```python
from build123d import *

# Parameters (mm, degrees)
SKETCH2_R               = 20
SKETCH2_R_2             = 4
BOSS_EXTRUDE1_DEPTH     = 21
CUT_EXTRUDE2_REACH      = 79.672
SKETCH3_R               = 2.5
CUT_EXTRUDE3_REACH      = 79.672
CUT_EXTRUDE3_END_RADIUS = 20
SKETCH4_R               = 2


with BuildPart() as part:
    # Sketch1 → Revolve1 (revolve)
    with BuildSketch(Plane(origin=(0, 0, 0), x_dir=(0, 0, -1), z_dir=(1, 0, 0))):
        Polygon((0, 0), (0, 52), (4, 52), (4, 20), (25, 20), (25, 0), align=None)
    revolve(axis=Axis((0, 0, -25), (0, 0, 1)))

    # Sketch2 → Boss-Extrude1 (add)
    with BuildSketch(Plane.XY):
        with Locations(Location((0, 0, 0), (0, 0, 90))):
            Circle(SKETCH2_R)
        with Locations(Location((0, 0, 0), (0, 0, 180))):
            Circle(SKETCH2_R_2, mode=Mode.SUBTRACT)
    extrude(amount=BOSS_EXTRUDE1_DEPTH)

    # Sketch3 → Cut-Extrude2 (cut, up to next)
    with BuildSketch(Plane(origin=(0, 0, -4), x_dir=(-1, 0, 0), z_dir=(0, 0, -1)), mode=Mode.PRIVATE) as cut_extrude2_sk1:
        with Locations(Location((0, 40, 0), (0, 0, 90))):
            Circle(SKETCH3_R)
    cut_extrude2_tool1 = extrude(cut_extrude2_sk1.sketch, amount=-CUT_EXTRUDE2_REACH, mode=Mode.PRIVATE) & part.part
    # Sketch3 → Cut-Extrude2 (cut, up to next)
    with BuildSketch(Plane(origin=(0, 0, -4), x_dir=(-1, 0, 0), z_dir=(0, 0, -1)), mode=Mode.PRIVATE) as cut_extrude2_sk2:
        with Locations(Location((34.641016151, 20, 0), (0, 0, 90))):
            Circle(SKETCH3_R)
    cut_extrude2_tool2 = extrude(cut_extrude2_sk2.sketch, amount=-CUT_EXTRUDE2_REACH, mode=Mode.PRIVATE) & part.part
    # Sketch3 → Cut-Extrude2 (cut, up to next)
    with BuildSketch(Plane(origin=(0, 0, -4), x_dir=(-1, 0, 0), z_dir=(0, 0, -1)), mode=Mode.PRIVATE) as cut_extrude2_sk3:
        with Locations(Location((34.641016151, -20, 0), (0, 0, 90))):
            Circle(SKETCH3_R)
    cut_extrude2_tool3 = extrude(cut_extrude2_sk3.sketch, amount=-CUT_EXTRUDE2_REACH, mode=Mode.PRIVATE) & part.part
    # Sketch3 → Cut-Extrude2 (cut, up to next)
    with BuildSketch(Plane(origin=(0, 0, -4), x_dir=(-1, 0, 0), z_dir=(0, 0, -1)), mode=Mode.PRIVATE) as cut_extrude2_sk4:
        with Locations(Location((0, -40, 0), (0, 0, 90))):
            Circle(SKETCH3_R)
    cut_extrude2_tool4 = extrude(cut_extrude2_sk4.sketch, amount=-CUT_EXTRUDE2_REACH, mode=Mode.PRIVATE) & part.part
    # Sketch3 → Cut-Extrude2 (cut, up to next)
    with BuildSketch(Plane(origin=(0, 0, -4), x_dir=(-1, 0, 0), z_dir=(0, 0, -1)), mode=Mode.PRIVATE) as cut_extrude2_sk5:
        with Locations(Location((-34.641016151, -20, 0), (0, 0, 90))):
            Circle(SKETCH3_R)
    cut_extrude2_tool5 = extrude(cut_extrude2_sk5.sketch, amount=-CUT_EXTRUDE2_REACH, mode=Mode.PRIVATE) & part.part
    # Sketch3 → Cut-Extrude2 (cut, up to next)
    with BuildSketch(Plane(origin=(0, 0, -4), x_dir=(-1, 0, 0), z_dir=(0, 0, -1)), mode=Mode.PRIVATE) as cut_extrude2_sk6:
        with Locations(Location((-34.641016151, 20, 0), (0, 0, 90))):
            Circle(SKETCH3_R)
    cut_extrude2_tool6 = extrude(cut_extrude2_sk6.sketch, amount=-CUT_EXTRUDE2_REACH, mode=Mode.PRIVATE) & part.part
    add(cut_extrude2_tool1.solids().sort_by_distance((0, 40, -4))[0], mode=Mode.SUBTRACT)
    add(cut_extrude2_tool2.solids().sort_by_distance((-34.641016, 20, -4))[0], mode=Mode.SUBTRACT)
    add(cut_extrude2_tool3.solids().sort_by_distance((-34.641016, -20, -4))[0], mode=Mode.SUBTRACT)
    add(cut_extrude2_tool4.solids().sort_by_distance((0, -40, -4))[0], mode=Mode.SUBTRACT)
    add(cut_extrude2_tool5.solids().sort_by_distance((34.641016, -20, -4))[0], mode=Mode.SUBTRACT)
    add(cut_extrude2_tool6.solids().sort_by_distance((34.641016, 20, -4))[0], mode=Mode.SUBTRACT)

    # Cut-Extrude3: up to this cylinder (the profile starts inside it)
    cut_extrude3_end = Plane(origin=(0, 0, 0), z_dir=(0, 0, -1)) * Cylinder(CUT_EXTRUDE3_END_RADIUS, 200.344, mode=Mode.PRIVATE)
    # Sketch4 → Cut-Extrude3 (cut, up to the surface)
    with BuildSketch(Plane(origin=(0, 0, 0), x_dir=(1, 0, 0), z_dir=(0, 1, 0)), mode=Mode.PRIVATE) as cut_extrude3_sk1:
        with Locations(Location((-10, 0, 0), (0, 0, 270))):
            Circle(SKETCH4_R)
    cut_extrude3_tool1 = extrude(cut_extrude3_sk1.sketch, amount=-CUT_EXTRUDE3_REACH, mode=Mode.PRIVATE) & cut_extrude3_end
    add(cut_extrude3_tool1.solids().sort_by_distance((-10, 0, 0))[0], mode=Mode.SUBTRACT)


solid = part.part
```
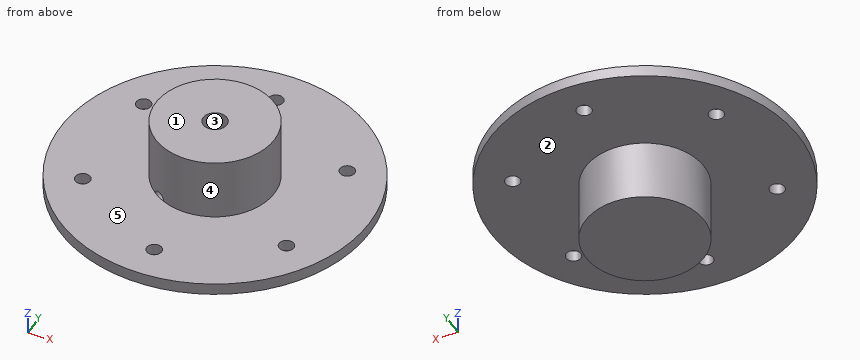
For this review, take the finished solid that the model builds, in its own axes (mm). Face numbers are marked on the shaded views. A direction names the side the tool comes from. Give positions to 0.01 mm unless a question says otherwise; leave off trailing zeros. Write each loop counter-clockwise with the first axis right and the second up, starting at its lowest first coordinate (ties: lowest second). Pieces come first, ordered by that corner, then holes. Notation, with made-up numbers: M -25.5,-24 L 23.5,-24 A27 ccw 23.5,7 Z; hole C -10.5,80.25 d2. An arc over 180 degrees is marked long. Answer as CSV lines item,"result".
1. Wall thickness on line 1 (X direction, y = -20, z = -1); line 2 (Z direction, x = 14, y = 34); line 3 (Y direction, x = -2.5, z = 1): over which ranges is each line inside the solid? List them lowest first.
Findings:
line 1,"x = -48 to -37.14, -32.14 to 32.14, 37.14 to 48"
line 2,"z = -4 to 0"
line 3,"y = -19.84 to -3.12, 3.12 to 19.84"
2. Consider section C-C, the plane y = -2. Write out the cut boundary in (x, z).
Findings:
outline,"M -51.96,-4 L -19.9,-4 L -19.9,-25 L 19.9,-25 L 19.9,-4 L 51.96,-4 L 51.96,0 L 19.9,0 L 19.9,21 L 3.46,21 L 3.46,0 L -3.46,0 L -3.46,21 L -19.9,21 L -19.9,0 L -51.96,0 Z; hole C -10,0 d4"
3. Consider section B-B, the plane y = 40. Write out the cut boundary in (x, z).
Findings:
outline,"M -33.23,-4 L -2.5,-4 L -2.5,0 L -33.23,0 Z; M 2.5,-4 L 33.23,-4 L 33.23,0 L 2.5,0 Z"
4. For pin 1 (1.5 mm diameter, centred on x = -13.5, y = -36, fed in from -Z); pin 2 (6.5 mm diameter, centred on x = 2, y = 1.5, fed in from +Z); pin 3 (6 mm diameter, centred on x = 0, y = -40, fed in from +Z); pin 4 (1 mm diameter, centred on y = 3, z = -13.5, fed in from +X), all flat-tipped, find the tip position at first contact; note any pin that passes through.
Findings:
pin 1,"stops at z = -4"
pin 2,"stops at z = 21"
pin 3,"stops at z = 0"
pin 4,"stops at x = 19.84"
5. Consider section A-A, the plane x = 0. Write out the cut boundary in (y, z).
Findings:
outline,"M -52,-4 L -42.5,-4 L -42.5,0 L -52,0 Z; M -37.5,-4 L -20,-4 L -20,-25 L 20,-25 L 20,-4 L 37.5,-4 L 37.5,0 L 20,0 L 20,21 L 4,21 L 4,0 L -4,0 L -4,21 L -20,21 L -20,0 L -37.5,0 Z; M 42.5,-4 L 52,-4 L 52,0 L 42.5,0 Z"
6. Draft analysis for pull direction X (two halves, no side actions). For the marked faces 3, 4 and 5, state which applies: +X half, -X half, draft (parallel to the pull), parting line (faces both ways), or undercut.
Findings:
face 3,"undercut"
face 4,"parting line"
face 5,"draft"
7. For the marked faces 1 and 2, list the 3-axis set-ups (+Z, -Z, +X, -X, +Y, -Y) from which the entire face can be reached by the end or side of a thin tool; tool diameter is ignored.
Findings:
face 1,"+Z, +X, -X, +Y, -Y"
face 2,"-Z"
8. Consider section D-D, the plane z = 11.5. Write out the cut boundary in (x, y).
Findings:
outline,"C 0,0 d40; hole C 0,0 d8"
